CAD build for the part. Positions are in the model's coordinates, mm. A direction names the side the tool comes from. Give positions to 0.01 mm unless a question says otherwise; leave off trailing zeros. Write each loop counter-clockwise with the first axis right and the second up, starting at its lowest first coordinate (ties: lowest second). Pieces come first, ordered by that corner, then holes. Notation, with made-up numbers: M 87.25,-30 L 107.25,-30 A21 cw 107.25,-4 Z; hole C -17,47 d6. An arc over 180 degrees is marked long. One line per question, with ' | ' between items. Start each with the question number.
1. Cut at A-A, the plane z = -6.5. Write the cut outline in (x, y).
2. Cut at D-D, the plane z = -1.5. Write the cut outline in (x, y), then the cut area to 3 significant figures.
3. Wall check: L1, parallel to X at y = -31, z = 9.5; L2, parallel to Y at x = -1.5, z = -3; L3, parallel to Z at x = -2.5, y = -44.5. Give the ranges that are in metal, low to high.
4. Which spindle directions (+Z, -Z, +X, -X, +Y, -Y) get a long thin tool onto all of the face, cutting with end or side? Do faces 4 (the face through (11, -44, 0)), 5 (the face through (31.732, -32.084, 8.458)), 6 (the face through (11.31, -64.03, -20.85)). Say none if no direction does.
5. Flat gauge pins, fed straight in: pin 1 (10 mm diameter, centred on x = 26.5, z = -7.5, fed in from +Y); pin 2 (2 mm diameter, centred on x = -4.15, y = -31, fed in from -Z); pin 3 (8 mm diameter, centred on y = -34, z = -3, fed in from +X); pin 4 (1 mm diameter, centred on x = 22.5, y = -55.5, fed in from -Z). Where does each tip first touch, or does it go through?
6. Cut at B-B, the plane y = -31. Write the cut outline in (x, z), then the cut area to 3 significant figures.
7. Pull direction Y, two halves, no side cores. Call faces 1 (the face through (-9.145, -30.78, 8.458)), 2 (the face through (8, -62, -12)), 3 (the face through (28.6, -30.92, 6.9)): released by +Y, released by -Y, zero draft, split by the parting line, or undercut.
8. Cut at C-C, the plane x = 16.5. Write the cut outline in (y, z).
```python
from build123d import *

# Parameters (mm, degrees)
F1_DEPTH = 4
F2_DEPTH = 14
F3_DEPTH = 30
F4_W     = 31
F4_H     = 4
F5_DEPTH = 24
F8_DEPTH = 25
F7_R     = 1.85
F9_DEPTH = 25


with BuildPart() as f1:
    # F0 (on Top) → F1 (new body)
    with BuildSketch(Plane.XY):
        with BuildLine():
            ThreePointArc((-4.1493639073, -29.25), (-2.9119270402, -29.7625631329), (-2.3993639073, -31))
            Line((-2.3993639073, -31), (0.8506360927, -31))
            ThreePointArc((0.8506360927, -31), (-0.6138300013, -27.4644660941), (-4.1493639073, -26))
            Line((-4.1493639073, -26), (-4.1493639073, -29.25))
        make_face()
        with BuildLine():
            Line((0.8506360927, -31), (-2.3993639073, -31))
            ThreePointArc((-2.3993639073, -31), (-5.3868007743, -32.2374368671), (-4.1493639073, -29.25))
            Line((-4.1493639073, -29.25), (-4.1493639073, -26))
            ThreePointArc((-4.1493639073, -26), (-9.1493639073, -31), (-4.1493639073, -36))
            ThreePointArc((-4.1493639073, -36), (-0.6138300013, -34.5355339059), (0.8506360927, -31))
        make_face()
        with BuildLine():
            ThreePointArc((-4.1493639073, -26), (-0.6138300013, -27.4644660941), (0.8506360927, -31))
            Line((0.8506360927, -31), (21.8506360927, -31))
            ThreePointArc((21.8506360927, -31), (23.3151021868, -27.4644660941), (26.8506360927, -26))
            Line((26.8506360927, -26), (18.1329660759, -26))
            ThreePointArc((18.1329660759, -26), (11.3506360927, -28), (4.5683061096, -26))
            Line((4.5683061096, -26), (-4.1493639073, -26))
        make_face()
        with BuildLine():
            ThreePointArc((26.8506360927, -26), (23.3151021868, -27.4644660941), (21.8506360927, -31))
            Line((21.8506360927, -31), (25.1006360927, -31))
            ThreePointArc((25.1006360927, -31), (25.6131992257, -29.7625631329), (26.8506360927, -29.25))
            Line((26.8506360927, -29.25), (26.8506360927, -26))
        make_face()
        with BuildLine():
            Line((25.1006360927, -31), (21.8506360927, -31))
            ThreePointArc((21.8506360927, -31), (23.3151021868, -34.5355339059), (26.8506360927, -36))
            ThreePointArc((26.8506360927, -36), (30.3861699987, -34.5355339059), (31.8506360927, -31))
            ThreePointArc((31.8506360927, -31), (30.3861699987, -27.4644660941), (26.8506360927, -26))
            Line((26.8506360927, -26), (26.8506360927, -29.25))
            ThreePointArc((26.8506360927, -29.25), (28.0880729598, -29.7625631329), (28.6006360927, -31))
            ThreePointArc((28.6006360927, -31), (26.8506360927, -32.75), (25.1006360927, -31))
        make_face()
        with BuildLine():
            Line((21.8506360927, -31), (0.8506360927, -31))
            ThreePointArc((0.8506360927, -31), (-0.6138300013, -34.5355339059), (-4.1493639073, -36))
            Line((-4.1493639073, -36), (26.8506360927, -36))
            ThreePointArc((26.8506360927, -36), (23.3151021868, -34.5355339059), (21.8506360927, -31))
        make_face()
    extrude(amount=F1_DEPTH)

    # F0 (on Top) → F2 (join)
    with BuildSketch(Plane.XY):
        with BuildLine():
            ThreePointArc((-4.1493639073, -29.25), (-2.9119270402, -29.7625631329), (-2.3993639073, -31))
            Line((-2.3993639073, -31), (0.8506360927, -31))
            ThreePointArc((0.8506360927, -31), (-0.6138300013, -27.4644660941), (-4.1493639073, -26))
            Line((-4.1493639073, -26), (-4.1493639073, -29.25))
        make_face()
        with BuildLine():
            Line((0.8506360927, -31), (-2.3993639073, -31))
            ThreePointArc((-2.3993639073, -31), (-5.3868007743, -32.2374368671), (-4.1493639073, -29.25))
            Line((-4.1493639073, -29.25), (-4.1493639073, -26))
            ThreePointArc((-4.1493639073, -26), (-9.1493639073, -31), (-4.1493639073, -36))
            ThreePointArc((-4.1493639073, -36), (-0.6138300013, -34.5355339059), (0.8506360927, -31))
        make_face()
        with BuildLine():
            ThreePointArc((26.8506360927, -26), (23.3151021868, -27.4644660941), (21.8506360927, -31))
            Line((21.8506360927, -31), (25.1006360927, -31))
            ThreePointArc((25.1006360927, -31), (25.6131992257, -29.7625631329), (26.8506360927, -29.25))
            Line((26.8506360927, -29.25), (26.8506360927, -26))
        make_face()
        with BuildLine():
            Line((25.1006360927, -31), (21.8506360927, -31))
            ThreePointArc((21.8506360927, -31), (23.3151021868, -34.5355339059), (26.8506360927, -36))
            ThreePointArc((26.8506360927, -36), (30.3861699987, -34.5355339059), (31.8506360927, -31))
            ThreePointArc((31.8506360927, -31), (30.3861699987, -27.4644660941), (26.8506360927, -26))
            Line((26.8506360927, -26), (26.8506360927, -29.25))
            ThreePointArc((26.8506360927, -29.25), (28.0880729598, -29.7625631329), (28.6006360927, -31))
            ThreePointArc((28.6006360927, -31), (26.8506360927, -32.75), (25.1006360927, -31))
        make_face()
    extrude(amount=F2_DEPTH)

    # F3 (add): a face of the model
    f3_faces = [f1.faces().sort_by_distance(p)[0] for p in [
        (11.3506360927, -36, 2),
    ]]
    extrude(f3_faces, amount=F3_DEPTH)

    # F4 (on face) → F5 (join)
    with BuildSketch(Plane(origin=(0, 0, 0), x_dir=(1, 0, 0), z_dir=(0, 0, -1))):
        with Locations((11.3506360927, 64)):
            Rectangle(F4_W, F4_H)
    extrude(amount=F5_DEPTH)

    # F6 (on face) → F8 (cut)
    with BuildSketch(Plane.XZ.offset(66)):
        with BuildLine():
            Line((13.2006360927, -19), (13.2006360927, -12))
            Line((13.2006360927, -12), (13.2006360927, -5))
            ThreePointArc((13.2006360927, -5), (11.3506360927, -3.15), (9.5006360927, -5))
            Line((9.5006360927, -5), (9.5006360927, -12))
            Line((9.5006360927, -12), (9.5006360927, -19))
            ThreePointArc((9.5006360927, -19), (11.3506360927, -20.85), (13.2006360927, -19))
        make_face()
    extrude(amount=-F8_DEPTH, mode=Mode.SUBTRACT)

    # F7 (on face) → F9 (cut)
    with BuildSketch(Plane.XY.offset(4)):
        with Locations((11.3506360927, -52)):
            Circle(F7_R)
    extrude(amount=-F9_DEPTH, mode=Mode.SUBTRACT)


solid = f1.part
```
Here are the results:
1) outline: M -4.15,-66 L 9.5,-66 L 9.5,-62 L -4.15,-62 Z; M 13.2,-66 L 26.85,-66 L 26.85,-62 L 13.2,-62 Z
2) outline: M -4.15,-66 L 26.85,-66 L 26.85,-62 L -4.15,-62 Z | area: 124 mm^2
3) L1: -9.15 to -5.9, -2.4 to 0.85, 21.85 to 25.1, 28.6 to 31.85 | L2: -66 to -62 | L3: 0 to 4
4) face 4: -Z, +X, -X, +Y | face 5: +Z | face 6: +Y, -Y
5) pin 1: y = -62 | pin 2: through | pin 3: x = 31.84 | pin 4: z = 0
6) outline: M -9.15,0 L -5.9,0 L -5.9,14 L -9.15,14 Z; M -2.4,0 L 25.1,0 L 25.1,14 L 21.85,14 L 21.85,4 L 0.85,4 L 0.85,14 L -2.4,14 Z; M 28.6,0 L 31.85,0 L 31.85,14 L 28.6,14 Z | area: 266 mm^2
7) face 1: split by the parting line | face 2: released by +Y | face 3: undercut
8) outline: M -66,-24 L -62,-24 L -62,0 L -26.89,0 L -26.89,4 L -66,4 Z
